Source: CAD feature listing. Evaluate the final solid. Frame: model axes, mm. Face numbers are marked on the shaded views. Coordinates: 2 decimals unless noted, no trailing zeros. Order: outer loops, then holes, each group sorted by start corner. A loop starts at its lowest first (then second) coordinate and runs counter-clockwise, first axis right, second up.
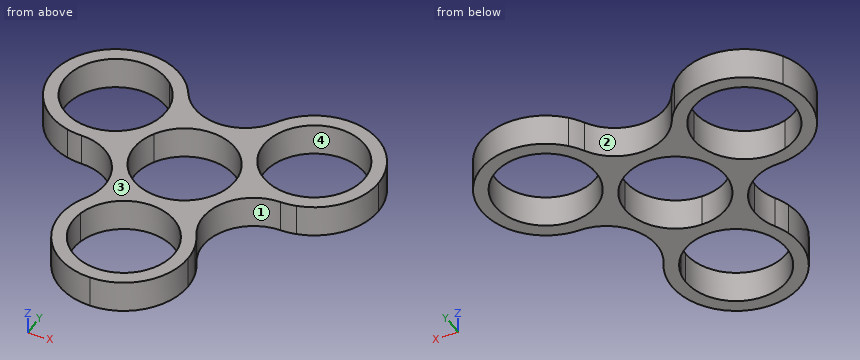
```python
from build123d import *

# Parameters (mm, degrees)
F1_DEPTH = 7


# Not quite as in the source:
# - a feature names something its author has since deleted; it is built from what else it names


with BuildPart() as f1:
    # F0 (on Top) → F1 (new body)
    with BuildSketch(Plane.XY):
        with BuildLine():
            ThreePointArc((9.5262796516, 5.4999996362), (10.6251841435, 2.8470092933), (11, 0))
            ThreePointArc((11, 0), (7.7781745931, -7.7781745931), (0, -11))
            ThreePointArc((0, -11), (6.9999999972, -12.8756443454), (12.1243556497, -17.9999999943))
            ThreePointArc((12.1243556497, -17.9999999943), (12.1243556546, -6.9999999972), (21.6506350946, -1.5))
            ThreePointArc((21.6506350946, -1.5), (14.6506352765, 0.375644242), (9.5262796516, 5.4999996362))
        make_face()
        with BuildLine():
            ThreePointArc((-9.5262796375, 5.4999996607), (1.41e-08, 11), (9.5262796516, 5.4999996362))
            ThreePointArc((9.5262796516, 5.4999996362), (7.6506350946, 12.4999999615), (9.5262796131, 19.500000297))
            ThreePointArc((9.5262796131, 19.500000297), (-4.54e-08, 14), (-9.5262796585, 19.5000003756))
            ThreePointArc((-9.5262796585, 19.5000003756), (-8.1276735827, 16.1234668409), (-7.6506350946, 12.5))
            ThreePointArc((-7.6506350946, 12.5), (-8.1276735773, 8.8765331793), (-9.5262796375, 5.4999996607))
        make_face()
        with BuildLine():
            ThreePointArc((9.5262796131, 19.500000297), (7.6506350946, 12.4999999615), (9.5262796516, 5.4999996362))
            ThreePointArc((9.5262796516, 5.4999996362), (14.6506352765, 0.375644242), (21.6506350946, -1.5))
            ThreePointArc((21.6506350946, -1.5), (23.3252484864, -1.3994845224), (24.9758155118, -1.0993814269))
            ThreePointArc((24.9758155118, -1.0993814269), (24.9939531467, -0.5498237016), (25, 0))
            ThreePointArc((25, 0), (24.9800177424, 0.9993565887), (24.9201029127, 1.9971156254))
            ThreePointArc((24.9201029127, 1.9971156254), (12.124355653, 7), (14.1896043222, 20.5828843746))
            ThreePointArc((14.1896043222, 20.5828843746), (12.8874554167, 21.4222662872), (11.5358155118, 22.1793814269))
            ThreePointArc((11.5358155118, 22.1793814269), (10.4506351975, 20.9000001372), (9.5262796131, 19.500000297))
        make_face()
        with BuildLine():
            ThreePointArc((-12.1243556177, -17.999999939), (-6.9999999695, -12.8756443294), (0, -11))
            ThreePointArc((0, -11), (-9.5262793437, -5.5000001697), (-9.5262796375, 5.4999996607))
            ThreePointArc((-9.5262796375, 5.4999996607), (-14.6506352643, 0.3756442491), (-21.6506350946, -1.5))
            ThreePointArc((-21.6506350946, -1.5), (-13.8724605016, -4.7218254069), (-10.6506350946, -12.5))
            ThreePointArc((-10.6506350946, -12.5), (-11.0254509963, -15.3470094621), (-12.1243556177, -17.999999939))
        make_face()
        with BuildLine():
            ThreePointArc((12.1243556497, -17.9999999943), (6.9999999972, -12.8756443454), (0, -11))
            ThreePointArc((0, -11), (-6.9999999695, -12.8756443294), (-12.1243556177, -17.999999939))
            ThreePointArc((-12.1243556177, -17.999999939), (-12.8746133779, -19.5005154452), (-13.44, -21.08))
            ThreePointArc((-13.44, -21.08), (-12.108499103, -21.8719969247), (-10.7304985905, -22.58))
            ThreePointArc((-10.7304985905, -22.58), (0, -14), (10.7304985905, -22.58))
            ThreePointArc((10.7304985905, -22.58), (12.108499103, -21.8719969247), (13.44, -21.08))
            ThreePointArc((13.44, -21.08), (12.8746133905, -19.5005154746), (12.1243556497, -17.9999999943))
        make_face()
        with BuildLine():
            ThreePointArc((-21.6506350946, -1.5), (-14.6506352643, 0.3756442491), (-9.5262796375, 5.4999996607))
            ThreePointArc((-9.5262796375, 5.4999996607), (-8.1276735773, 8.8765331793), (-7.6506350946, 12.5))
            ThreePointArc((-7.6506350946, 12.5), (-8.1276735827, 16.1234668409), (-9.5262796585, 19.5000003756))
            ThreePointArc((-9.5262796585, 19.5000003756), (-10.4506352247, 20.9000001735), (-11.5358155118, 22.1793814269))
            ThreePointArc((-11.5358155118, 22.1793814269), (-12.8874554167, 21.4222662872), (-14.1896043222, 20.5828843746))
            ThreePointArc((-14.1896043222, 20.5828843746), (-11.5741441752, 16.9118398375), (-10.6506350946, 12.5))
            ThreePointArc((-10.6506350946, 12.5), (-15.1300578962, 3.6409891636), (-24.9201029127, 1.9971156254))
            ThreePointArc((-24.9201029127, 1.9971156254), (-24.9959545198, 0.4497306374), (-24.9758155118, -1.0993814269))
            ThreePointArc((-24.9758155118, -1.0993814269), (-23.3252484864, -1.3994845224), (-21.6506350946, -1.5))
        make_face()
        with BuildLine():
            ThreePointArc((33.7749911327, 19.499999333), (23.3252488687, 26.3994844763), (11.5358155118, 22.1793814269))
            ThreePointArc((11.5358155118, 22.1793814269), (12.8874554167, 21.4222662872), (14.1896043222, 20.5828843746))
            ThreePointArc((14.1896043222, 20.5828843746), (26.0624749321, 22.5764909194), (32.6506350946, 12.5))
            ThreePointArc((32.6506350946, 12.5), (30.509645931, 5.9794228016), (24.9201029127, 1.9971156254))
            ThreePointArc((24.9201029127, 1.9971156254), (24.9800177424, 0.9993565887), (25, 0))
            ThreePointArc((25, 0), (24.9939531467, -0.5498237016), (24.9758155118, -1.0993814269))
            ThreePointArc((24.9758155118, -1.0993814269), (32.6631853406, 3.8557107244), (35.6506350946, 12.5))
            ThreePointArc((35.6506350946, 12.5), (35.1735967623, 16.1234662595), (33.7749911327, 19.499999333))
        make_face()
        with BuildLine():
            ThreePointArc((14, -25), (13.8592929113, -23.0201010127), (13.44, -21.08))
            ThreePointArc((13.44, -21.08), (12.108499103, -21.8719969247), (10.7304985905, -22.58))
            ThreePointArc((10.7304985905, -22.58), (10.9324170359, -23.782519917), (11, -25))
            ThreePointArc((11, -25), (-1.217480083, -35.9324170359), (-10.7304985905, -22.58))
            ThreePointArc((-10.7304985905, -22.58), (-12.108499103, -21.8719969247), (-13.44, -21.08))
            ThreePointArc((-13.44, -21.08), (-11.2000000155, -33.3999999793), (-5.18e-08, -39))
            ThreePointArc((-5.18e-08, -39), (9.8994949183, -34.8994949549), (14, -25))
        make_face()
        with BuildLine():
            ThreePointArc((-33.7749911175, 19.4999993593), (-34.5252483411, 7.0005151375), (-24.9758155118, -1.0993814269))
            ThreePointArc((-24.9758155118, -1.0993814269), (-24.9959545198, 0.4497306374), (-24.9201029127, 1.9971156254))
            ThreePointArc((-24.9201029127, 1.9971156254), (-31.1769145362, 18), (-14.1896043222, 20.5828843746))
            ThreePointArc((-14.1896043222, 20.5828843746), (-12.8874554167, 21.4222662872), (-11.5358155118, 22.1793814269))
            ThreePointArc((-11.5358155118, 22.1793814269), (-23.3252488536, 26.3994844781), (-33.7749911175, 19.4999993593))
        make_face()
    extrude(amount=F1_DEPTH)


solid = f1.part
```
1. Section query B-B on y = -19. Return loops of the section in (x, z), plus the area to 3 significant figures.
Findings:
outline: (-12.65, 0) - (-9.22, 0) - (-9.22, 7) - (-12.65, 7) - close; (9.22, 0) - (12.65, 0) - (12.65, 7) - (9.22, 7) - close
area: 48.0 mm2
2. Section query A-A on x = -19.5. Return loops of the section in (y, z), plus the area to 3 significant figures.
Findings:
outline: (-1.71, 0) - (1.71, 0) - (1.71, 7) - (-1.71, 7) - close; (23.29, 0) - (26.33, 0) - (26.33, 7) - (23.29, 7) - close
area: 45.3 mm2
3. Section query D-D on z = 1.5. Return loops of the section in (x, y) (1 decimal).
Findings:
outline: (-21.7, -1.5) arc R11 cw to (-12.1, -18) arc R14 ccw (long way) to (12.1, -18) arc R11 cw to (21.7, -1.5) arc R14 ccw (long way) to (9.5, 19.5) arc R11 cw to (-9.5, 19.5) arc R14 ccw (long way) to start; hole circle Ø22 at (-21.7, 12.5); hole circle Ø22 at (0, -25); hole circle Ø22 at (0, 0); hole circle Ø22 at (21.7, 12.5)
4. Section query C-C on x = 7.5. Return loops of the section in (y, z), plus the area to 3 significant figures.
Findings:
outline: (-36.82, 0) - (-33.05, 0) - (-33.05, 7) - (-36.82, 7) - close; (-16.95, 0) - (-8.05, 0) - (-8.05, 7) - (-16.95, 7) - close; (8.05, 0) - (16.95, 0) - (16.95, 7) - (8.05, 7) - close
area: 151 mm2
5. Draft query along X for the marked faces 1, 2, 3 and 4. Return one class per face: released by +X, released by -X, zero draft, split by the parting line, or undercut.
Findings:
face 1: released by +X
face 2: undercut
face 3: zero draft
face 4: undercut
6. Pin query (flat end, axial travel): P1, Ø1.5, axis at x = -9.5, y = -14, coming from the -Z side; P2, Ø1, axis at x = 17.5, z = 5.5, coming from the -Y side; P3, Ø4, axis at y = -28.5, z = 3, coming from the +X side; P4, Ø3, axis at y = -20, z = 4, coming from the -X side. Return the tip coordinate at first contact, or that it passes through.
Findings:
P1: stops at z = 0
P2: stops at y = -2.53
P3: stops at x = 13.92
P4: stops at x = -13.56
7. Ray query, line 1 (X direction, y = 12.5, z = 2.75); line 2 (X direction, y = -25, z = 2.75); line 3 (X direction, y = 20.5, z = 2.25). Return the intervals inside material, ascending.
Findings:
line 1: x = -35.65 to -32.65, -10.65 to 10.65, 32.65 to 35.65
line 2: x = -14 to -11, 11 to 14
line 3: x = -33.14 to -29.2, -14.1 to -10.16, 10.16 to 14.1, 29.2 to 33.14
